Source: CAD feature listing. Evaluate the final solid. Frame: model axes, mm. Face numbers are marked on the shaded views. A direction names the side the tool comes from. Give positions to 0.01 mm unless a question says otherwise; leave off trailing zeros. Loops run counter-clockwise (first coordinate to the right, second up) from the corner with the lowest first, then second, coordinate; pieces in that order, holes last. Notation, with made-up numbers: M 46,77 L 57,77 A12 ccw 57,93 Z; hole C -24.75,74.5 d9. An arc over 180 degrees is marked long. Write item = value, one per line.
from build123d import *

# Parameters (mm, degrees)
F1_DEPTH = 25


with BuildPart() as f1:
    # F0 (on Front) → F1 (new body)
    with BuildSketch(Plane.XZ):
        with BuildLine():
            Line((-2.425778, 4.31487), (-5.591055, 9.240136))
            ThreePointArc((-5.591055, 9.240136), (-5.838921, 9.085538), (-6.082515, 8.924293))
            Line((-6.082515, 8.924293), (-2.917239, 3.999027))
            ThreePointArc((-2.917239, 3.999027), (-3.241561, 3.74096), (-3.543157, 3.456666))
            Line((-3.543157, 3.456666), (-7.967825, 7.290663))
            ThreePointArc((-7.967825, 7.290663), (-8.162095, 7.072496), (-8.350394, 6.849154))
            Line((-8.350394, 6.849154), (-3.925726, 3.015157))
            ThreePointArc((-3.925726, 3.015157), (-4.164205, 2.676172), (-4.373489, 2.318424))
            Line((-4.373489, 2.318424), (-9.699089, 4.750544))
            ThreePointArc((-9.699089, 4.750544), (-9.824026, 4.486482), (-9.941774, 4.219137))
            Line((-9.941774, 4.219137), (-4.616175, 1.787017))
            ThreePointArc((-4.616175, 1.787017), (-4.74949, 1.394576), (-4.849508, 0.992358))
            Line((-4.849508, 0.992358), (-10.644591, 1.825565))
            ThreePointArc((-10.644591, 1.825565), (-10.690072, 1.537), (-10.727731, 1.247311))
            Line((-10.727731, 1.247311), (-4.932648, 0.414104))
            ThreePointArc((-4.932648, 0.414104), (-4.95, 0), (-4.932648, -0.414104))
            Line((-4.932648, -0.414104), (-10.727731, -1.247311))
            ThreePointArc((-10.727731, -1.247311), (-10.690072, -1.537), (-10.644591, -1.825565))
            Line((-10.644591, -1.825565), (-4.849508, -0.992358))
            ThreePointArc((-4.849508, -0.992358), (-4.74949, -1.394576), (-4.616175, -1.787017))
            Line((-4.616175, -1.787017), (-9.941774, -4.219137))
            ThreePointArc((-9.941774, -4.219137), (-9.824026, -4.486482), (-9.699089, -4.750544))
            Line((-9.699089, -4.750544), (-4.373489, -2.318424))
            ThreePointArc((-4.373489, -2.318424), (-4.164205, -2.676172), (-3.925726, -3.015157))
            Line((-3.925726, -3.015157), (-8.350394, -6.849154))
            ThreePointArc((-8.350394, -6.849154), (-8.162095, -7.072496), (-7.967825, -7.290663))
            Line((-7.967825, -7.290663), (-3.543157, -3.456666))
            ThreePointArc((-3.543157, -3.456666), (-3.241561, -3.74096), (-2.917239, -3.999027))
            Line((-2.917239, -3.999027), (-6.082515, -8.924293))
            ThreePointArc((-6.082515, -8.924293), (-5.838921, -9.085538), (-5.591055, -9.240136))
            Line((-5.591055, -9.240136), (-2.425778, -4.31487))
            ThreePointArc((-2.425778, -4.31487), (-2.056304, -4.502678), (-1.672414, -4.65892))
            Line((-1.672414, -4.65892), (-3.321866, -10.276439))
            ThreePointArc((-3.321866, -10.276439), (-2.702728, -10.45635), (-2.073957, -10.598995))
            Line((-2.073957, -10.598995), (1.778874, -10.652493))
            ThreePointArc((1.778874, -10.652493), (2.557292, -10.492867), (3.321866, -10.276439))
            Line((3.321866, -10.276439), (1.672414, -4.65892))
            ThreePointArc((1.672414, -4.65892), (2.056304, -4.502678), (2.425778, -4.31487))
            Line((2.425778, -4.31487), (5.591055, -9.240136))
            ThreePointArc((5.591055, -9.240136), (5.838921, -9.085538), (6.082515, -8.924293))
            Line((6.082515, -8.924293), (2.917239, -3.999027))
            ThreePointArc((2.917239, -3.999027), (3.241561, -3.74096), (3.543157, -3.456666))
            Line((3.543157, -3.456666), (7.967825, -7.290663))
            ThreePointArc((7.967825, -7.290663), (8.162095, -7.072496), (8.350394, -6.849154))
            Line((8.350394, -6.849154), (3.925726, -3.015157))
            ThreePointArc((3.925726, -3.015157), (4.164205, -2.676172), (4.373489, -2.318424))
            Line((4.373489, -2.318424), (9.699089, -4.750544))
            ThreePointArc((9.699089, -4.750544), (9.824026, -4.486482), (9.941774, -4.219137))
            Line((9.941774, -4.219137), (4.616175, -1.787017))
            ThreePointArc((4.616175, -1.787017), (4.74949, -1.394576), (4.849508, -0.992358))
            Line((4.849508, -0.992358), (10.644591, -1.825565))
            ThreePointArc((10.644591, -1.825565), (10.690072, -1.537), (10.727731, -1.247311))
            Line((10.727731, -1.247311), (4.932648, -0.414104))
            ThreePointArc((4.932648, -0.414104), (4.95, 0), (4.932648, 0.414104))
            Line((4.932648, 0.414104), (10.727731, 1.247311))
            ThreePointArc((10.727731, 1.247311), (10.690072, 1.537), (10.644591, 1.825565))
            Line((10.644591, 1.825565), (4.849508, 0.992358))
            ThreePointArc((4.849508, 0.992358), (4.74949, 1.394576), (4.616175, 1.787017))
            Line((4.616175, 1.787017), (9.941774, 4.219137))
            ThreePointArc((9.941774, 4.219137), (9.824026, 4.486482), (9.699089, 4.750544))
            Line((9.699089, 4.750544), (4.373489, 2.318424))
            ThreePointArc((4.373489, 2.318424), (4.164205, 2.676172), (3.925726, 3.015157))
            Line((3.925726, 3.015157), (8.350394, 6.849154))
            ThreePointArc((8.350394, 6.849154), (8.162095, 7.072496), (7.967825, 7.290663))
            Line((7.967825, 7.290663), (3.543157, 3.456666))
            ThreePointArc((3.543157, 3.456666), (3.241561, 3.74096), (2.917239, 3.999027))
            Line((2.917239, 3.999027), (6.082515, 8.924293))
            ThreePointArc((6.082515, 8.924293), (5.838921, 9.085538), (5.591055, 9.240136))
            Line((5.591055, 9.240136), (2.425778, 4.31487))
            ThreePointArc((2.425778, 4.31487), (2.056304, 4.502678), (1.672414, 4.65892))
            Line((1.672414, 4.65892), (3.321866, 10.276439))
            ThreePointArc((3.321866, 10.276439), (2.720175, 10.451825), (2.109323, 10.592014))
            Line((2.109323, 10.592014), (-2.310303, 10.55))
            ThreePointArc((-2.310303, 10.55), (-2.819405, 10.425496), (-3.321866, 10.276439))
            Line((-3.321866, 10.276439), (-1.672414, 4.65892))
            ThreePointArc((-1.672414, 4.65892), (-2.056304, 4.502678), (-2.425778, 4.31487))
        make_face()
    extrude(amount=F1_DEPTH)


solid = f1.part
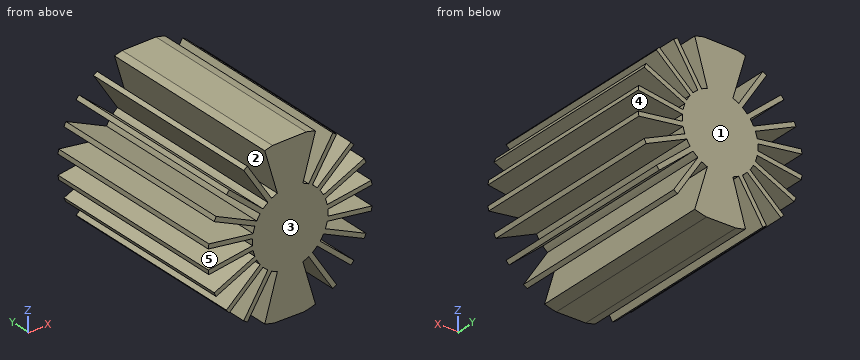
1. Cut plane A-A, the plane x = 9. Return the cut outline in (y, z).
Derived:
outline = M -25,-4.43 L 0,-4.43 L 0,-3.79 L -25,-3.79 Z; M -25,-1.59 L 0,-1.59 L 0,-1 L -25,-1 Z; M -25,1 L 0,1 L 0,1.59 L -25,1.59 Z; M -25,3.79 L 0,3.79 L 0,4.43 L -25,4.43 Z
2. First-contact query: pin 1 Ø6 at (y, z) = (-21, -8.5) entering from +X; pin 2 Ø10 at (y, z) = (-7.5, 8.5) entering from +X. Flat tips, straight axial feed; report the tip coordinate or a pass-through.
Derived:
pin_1 = 8.35
pin_2 = 9.94
3. Reachability of the marked faces 1, 2, 3, 4 and 5 from +Z, -Z, +X, -X, +Y, -Y: full face, straight path, thin tool, end or side. Return the list, or none.
Derived:
face_1 = +Z, -Z, +X, -X, +Y
face_2 = +Y, -Y
face_3 = +Z, -Z, +X, -X, -Y
face_4 = +X, +Y, -Y
face_5 = -X, +Y, -Y
4. Material intervals for probe 1 along X at (y, z) = (-8.5, 2.75); probe 2 along Z at (x, y) = (-7.75, -14.75); probe 3 along Z at (x, y) = (-4, -3.5), sorted ascending. Write a range as from..to.
Derived:
probe_1 = -6.72..-5.32, -4.12..4.12, 5.32..6.72
probe_2 = -7.1..-6.33, -3.86..-3.22, -1.41..-0.82, 0.82..1.41, 3.22..3.86, 6.33..7.1
probe_3 = -6.76..-5.68, -3.85..-3.08, -2.92..2.92, 3.08..3.85, 5.68..6.76
5. Cut plane B-B, the plane z = 7.75. Return the cut outline in (x, y), then the cut area to 3 significant figures.
Derived:
outline = M -5.33,-25 L -4.63,-25 L -4.63,0 L -5.33,0 Z; M -2.58,-25 L 2.58,-25 L 2.58,0 L -2.58,0 Z; M 4.63,-25 L 5.33,-25 L 5.33,0 L 4.63,0 Z
area = 164 mm²
